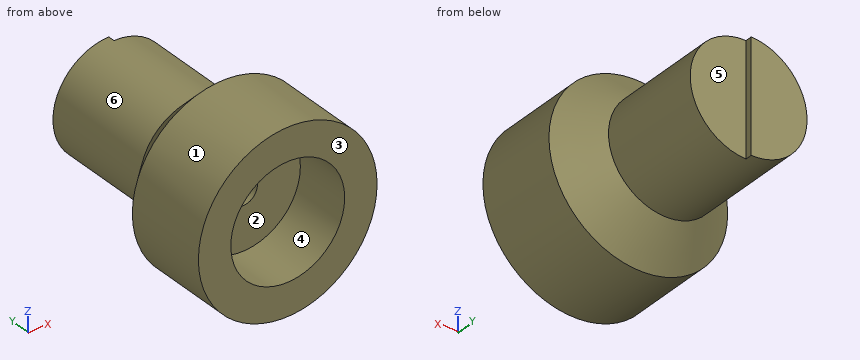
from build123d import *

# Parameters (mm, degrees)
SKETCH_4_W             = 5
SKETCH_4_H             = 10
CUT_EXTRUDE_849_DEPTH  = 0.6
CHAMFER_1_SIZE         = 3
SKETCH_5_R             = 5.1
CUT_EXTRUDE_1019_DEPTH = 5.1
HOLE_WIZARD_M3_D       = 2.5
HOLE_WIZARD_M3_DEPTH   = 10
HOLE_WIZARD_M3_TIP     = 0.751075774


with BuildPart() as part:
    # Эскиз1 → Revolve 497 (revolve)
    with BuildSketch(Plane.XY):
        Polygon((0, 10.3), (-5, 10.3), (-5, 0.3), (-8, 0.3), (-8, -10.3), (0, -10.3), align=None)
    revolve(axis=Axis((0, 10.3, 0), (0, -1, 0)))

    # Эскиз4 → Cut-Extrude 849 (cut)
    with BuildSketch(Plane(origin=(0, 10.3, 0), x_dir=(1, 0, 0), z_dir=(0, 1, 0))):
        with Locations((2.5, 0)):
            Rectangle(SKETCH_4_W, SKETCH_4_H)
    extrude(amount=-CUT_EXTRUDE_849_DEPTH, mode=Mode.SUBTRACT)

    # Фаска1
    chamfer_1_edges = [part.edges().sort_by_distance(p)[0] for p in [
        (8, 0.3, 0),
    ]]
    chamfer(chamfer_1_edges, length=CHAMFER_1_SIZE - 0.0001)  # a hair under: the kernel refuses the full size

    # Эскиз5 → Cut-Extrude 1019 (cut)
    with BuildSketch(Plane.XZ.offset(10.3)):
        Circle(SKETCH_5_R)
    extrude(amount=-CUT_EXTRUDE_1019_DEPTH, mode=Mode.SUBTRACT)

    # Крепление магнита M3
    with Locations(Plane(origin=(0, -5.2, 0), x_dir=(-1, 0, 0), z_dir=(0, -1, 0))):
        with Locations((0, 0)):
            Hole(HOLE_WIZARD_M3_D / 2, depth=HOLE_WIZARD_M3_DEPTH)
            with Locations((0, 0, -(HOLE_WIZARD_M3_DEPTH + HOLE_WIZARD_M3_TIP / 2))):  # 118° drill point
                Cone(0, HOLE_WIZARD_M3_D / 2, HOLE_WIZARD_M3_TIP, mode=Mode.SUBTRACT)


solid = part.part
For this review, take the finished solid that the model builds, in its own axes (mm). Face numbers are marked on the shaded views. A direction names the side the tool comes from. Round coordinates to 2 decimals unless told otherwise and drop trailing zeros. Order: outer loops, then holes, each group sorted by start corner. A loop starts at its lowest first (then second) coordinate and runs counter-clockwise, first axis right, second up. Notation, with made-up numbers: (4, 5) -> (33, 5) arc R20 cw to (33, 34) -> close; hole circle Ø9 at (-12, -29). An arc over 180 degrees is marked (long way). Write item = value, one per line. Start each with the question number.
1) To check wall thickness, follow line 1 (Z direction, x = 0, y = -7.45); line 2 (X direction, y = -5.5, z = -0.25); line 3 (Z direction, x = 0, y = 1.75). State the ranges of each line that lie inside material, in increasing order. Write a range as from..to.
2) Tool access review of the marked faces 4, 5 and 6: name each direction out of +Z, -Z, +X, -X, +Y, -Y from which nothing blocks a thin tool from reaching the whole face with its end or side.
3) The part is to be moulded in two halves that separate along Z. For the marked faces 1, 2 and 3, say which applies: +Z half, -Z half, draft (parallel to the pull), parting line (faces both ways), or undercut.
4) Insertion check: pin 1 (3 mm diameter, centred on x = 3, y = 7.5, fed in from -Z); pin 2 (3 mm diameter, centred on y = -7.5, z = 5.5, fed in from -X); pin 3 (0.5 mm diameter, centred on y = 10, z = 0, fed in from +X). Each pin has a flat end and moves straight along its axis. Give the tip position at first contact, or say it passes through.
5) Take a section at B-B on y = -7.5. State the section outline as (x, z) points, plus the area to 3 significant figures.
6) Take a section at A-A on y = -4.5. State the section outline as (x, z) points, plus the area to 3 significant figures.
Verdict:
q1.line_1 = -8..-5.1, 5.1..8
q1.line_2 = -8..-5.09, 5.09..8
q1.line_3 = -5..-1.25, 1.25..5
q2.face_4 = -Y
q2.face_5 = +Z, -Z, +X, +Y
q2.face_6 = +Y
q3.face_1 = parting line
q3.face_2 = undercut
q3.face_3 = draft
q4.pin_1 = -4.77
q4.pin_2 = -6.93
q4.pin_3 = 0
q5.outline = circle Ø16 at (0, 0); hole circle Ø10.2 at (0, 0)
q5.area = 119 mm2
q6.outline = circle Ø16 at (0, 0); hole circle Ø2.5 at (0, 0)
q6.area = 196 mm2
